```python
from build123d import *

# Parameters (mm, degrees)
F2_R           = 14.99999
F4_D           = 5
F4_CBORE_D     = 8
F4_CBORE_DEPTH = 2


# Not quite as in the source:
# - a fillet or chamfer is up to 0.001 mm smaller than in the source, because OpenCascade refuses the exact size


with BuildPart() as f1:
    # F0 (on Front) → F1 (revolve)
    with BuildSketch(Plane.XZ):
        Polygon((28, -25), (0, -25), (0, -30), (43, -30), (43, -15), (28, -15), align=None)
    revolve(axis=Axis((0, 0, -27.5), (0, 0, 1)))

    # F2 (radius 15 in the source; OpenCascade refuses exactly that, so slightly less here)
    f2_edges = [f1.edges().sort_by_distance(p)[0] for p in [
        (-43, 0, -30),
    ]]
    fillet(f2_edges, radius=F2_R)

    # F4 (through all)
    with Locations(Plane(origin=(0, 0, -30), x_dir=(1, 0, 0), z_dir=(0, 0, -1))):
        with Locations((-12.9903810568, 7.5), (12.9903810568, 7.5), (0, -15)):
            CounterBoreHole(F4_D / 2, F4_CBORE_D / 2, F4_CBORE_DEPTH)


solid = f1.part
```
Check sheet for the modelled part. Datum: model origin and axes. Units: mm. A direction names the side the tool comes from. Give positions to 0.01 mm unless a question says otherwise; leave off trailing zeros. Loops run counter-clockwise (first coordinate to the right, second up) from the corner with the lowest first, then second, coordinate; pieces in that order, holes last. Notation, with made-up numbers: (-23, 24.5) - (-7, 24.5) arc R34 cw to (-7, 55.5) - close; hole circle Ø7 at (-35, 44). An arc over 180 degrees is marked (long way). One line per question, with ' | ' between items. Start each with the question number.
1. Draft check along X on faces 1 (the cylindrical face through (9.816, -5.066, -29.014)), 2 (the flat face through (0, 0, -30)). Enter one of: released by +X, released by -X, zero draft, split by the parting line, or undercut.
2. Cross-section at D-D, the plane z = -18.75. Enter the section's corners in (x, y), plus the area to 3 significant figures.
3. Set-up check for faces 3 (the flat face through (9, -28, -15)), 4 (the flat face through (16, -8, -28)), 5 (the cylindrical face through (25.865, -10.724, -20.07)): record each of +Z, -Z, +X, -X, +Y, -Y from which the full face is reachable in a straight line by a thin tool's end or side.
4. Cross-section at C-C, the plane z = -27. Enter the section's corners in (x, y), plus the area to 3 significant figures.
5. Material ranges on line 1 along Z through (x, y) = (6, -16.5); line 2 along Y through (x, z) = (0, -19.5); line 3 along Y through (x, z) = (23, -19.75), recorded low to high. Write a range as [from, to].
6. Gauge pin test, flat ends, axial feed: pin 1 Ø8 at (x, y) = (12.99, -7.5) entering from +Z; pin 2 Ø6.5 at (x, y) = (0, 15) entering from -Z; pin 3 Ø1.5 at (x, z) = (-6, -17.5) entering from +Y. Record the tip position at first contact, or that the pin passes through.
Check result:
1) face 1: undercut | face 2: zero draft
2) outline: circle Ø85.05 at (0, 0); hole circle Ø56 at (0, 0) | area: 3,220 mm2
3) face 3: +Z, +X, -X, +Y, -Y | face 4: -Z | face 5: +Z
4) outline: circle Ø74 at (0, 0); hole circle Ø5 at (-12.99, -7.5); hole circle Ø5 at (0, 15); hole circle Ø5 at (12.99, -7.5) | area: 4,240 mm2
5) line 1: z = [-30, -25] | line 2: y = [-42.31, -28], [28, 42.31] | line 3: y = [-35.41, -15.97], [15.97, 35.41]
6) pin 1: stops at z = -25 | pin 2: stops at z = -28 | pin 3: stops at y = 42.52
